For this review, use the dimensioned drawing (mm, ordinates from the lowest corner) and the shaded views. Give positions to 0.01 mm unless a question says otherwise; leave off trailing zeros. Write each loop counter-clockwise with the first axis right and the second up, starting at its lowest first coordinate (ties: lowest second). Pieces come first, ordered by that corner, then holes. Notation, with made-up numbers: M -23,19.25 L 35,19.25 A15 ccw 35,38.25 Z; hole C -40,8 d8. An arc over 180 degrees is marked long. Use a Markdown table: item, result. Add a question column.
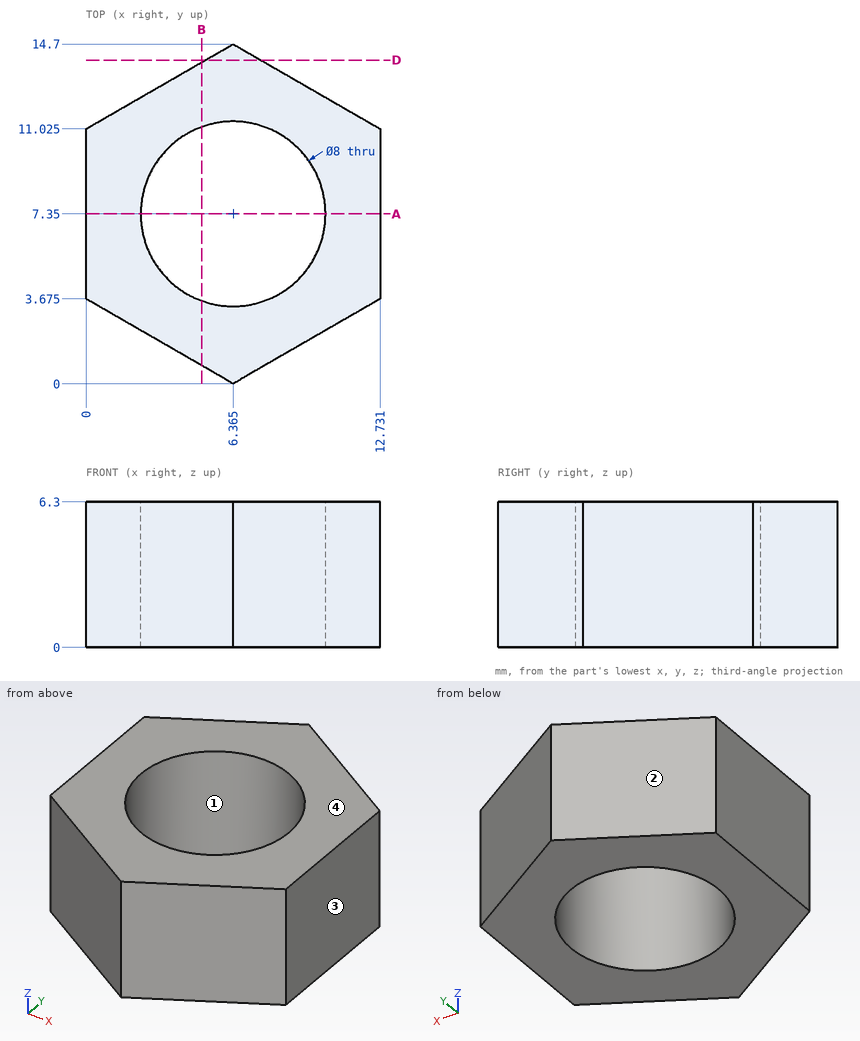
(1) For pin 1 (2 mm diameter, centred on x = 11.5, z = 2.5, fed in from +Y); pin 2 (7 mm diameter, centred on x = 6.37, y = 7.35, fed in from +Z); pin 3 (3 mm diameter, centred on x = 8.5, z = 4.5, fed in from +Y); pin 4 (1.5 mm diameter, centred on x = 11, z = 2, fed in from +Y), all flat-tipped, find the tip position at first contact; note any pin that passes through.
(2) Add section A-A on y = 7.35. Give the boundary of the cut face in (x, z) (1 decimal).
(3) Add section B-B on x = 5. Give the boundary of the cut face in (y, z).
(4) The part is to be moulded in two halves that separate along X. For the marked faces 1, 2, 3 and 4, say which applies: released by +X, released by -X, zero draft, split by the parting line, or undercut.
(5) Add section D-D on y = 14. Give the boundary of the cut face in (x, z), then the cut area to 3 significant figures.
(6) Wall thickness on L1, parallel to X at y = 7.35, z = 2.25 (1 decimal); L2, parallel to Y at x = 7, z = 5.5 (1 decimal); L3, parallel to X at y = 6, z = 2.25: over which ranges is each line inside the solid? List them lowest first.
From the geometry:
| question | item | result |
|---|---|---|
| 1 | pin 1 | stops at y = 12.31 |
| 1 | pin 2 | passes through |
| 1 | pin 3 | stops at y = 14.33 |
| 1 | pin 4 | stops at y = 12.46 |
| 2 | outline | M 0,0 L 2.4,0 L 2.4,6.3 L 0,6.3 Z; M 10.4,0 L 12.7,0 L 12.7,6.3 L 10.4,6.3 Z |
| 3 | outline | M 0.79,0 L 3.59,0 L 3.59,6.3 L 0.79,6.3 Z; M 11.11,0 L 13.91,0 L 13.91,6.3 L 11.11,6.3 Z |
| 4 | face 1 | undercut |
| 4 | face 2 | released by -X |
| 4 | face 3 | released by +X |
| 4 | face 4 | zero draft |
| 5 | outline | M 5.15,0 L 7.58,0 L 7.58,6.3 L 5.15,6.3 Z |
| 5 | area | 15.3 mm^2 |
| 6 | L1 | x = 0 to 2.4, 10.4 to 12.7 |
| 6 | L2 | y = 0.4 to 3.4, 11.3 to 14.3 |
| 6 | L3 | x = 0 to 2.6, 10.13 to 12.73 |
